Could you check a few things on this drawing? It's one solid part, dimensions in mm from its lowest x, y, z. A direction names the side the tool comes from. Give positions to 0.01 mm unless a question says otherwise; leave off trailing zeros. Loops run counter-clockwise (first coordinate to the right, second up) from the corner with the lowest first, then second, coordinate; pieces in that order, holes last. Notation, with made-up numbers: M 14.5,72.5 L 50.5,72.5 A33 ccw 50.5,106.5 Z; hole C 45.5,86.25 d10. An arc over 180 degrees is marked long. Return JSON: item names as keys, results as strings. Group by question number.
1. If we section it at A-A (z = 7.25): Write out the boundary of the cut face in (x, y), plus the area to 3 significant figures.
2. Please list where these lines run through material, in increasing order: line 1 (X direction, y = 19.5, z = 3.5); line 2 (Y direction, x = 36, z = 5.75); line 3 (Z direction, x = 38.5, y = 3.5).
3. If we mould it in two halves opening along Y, with no side actions, what happens to the marked faces 1, 2, 3 and 4? For each: +Y half, -Y half, draft (parallel to the pull), parting line (faces both ways), or undercut.
4. For the marked faces 5 and 6, which set-ups out of +Z, -Z, +X, -X, +Y, -Y let a thin tool reach every point of the face, with its end or its side?
5. If we section it at C-C (x = 17): Write out the boundary of the cut face in (y, z).
6. If we section it at B-B (y = 13.5): Write out the boundary of the cut face in (x, z).
7. For pin 1 (0.5 mm diameter, centred on x = 63, z = 0.5, fed in from -Y); pin 2 (0.7 mm diameter, centred on x = 63, z = 0, fed in from +Y); pin 3 (0.6 mm diameter, centred on x = 63, y = 15, fed in from -Z), each with a flat end and sliding along its axis, tell me the tip position at first contact or that it passes through.
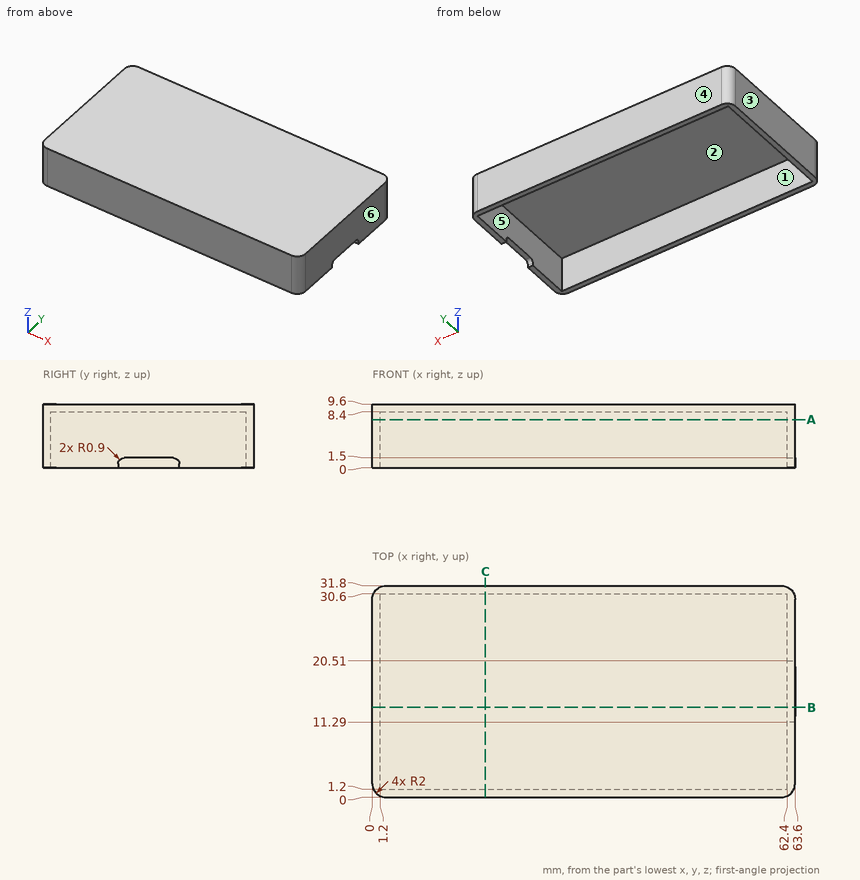
Answer:
{
 "1": {"outline": "M 0,2 A2 ccw 2,0 L 61.6,0 A2 ccw 63.6,2 L 63.6,29.8 A2 ccw 61.6,31.8 L 2,31.8 A2 ccw 0,29.8 Z; hole M 1.2,1.2 L 62.4,1.2 L 62.4,30.6 L 1.2,30.6 Z", "area": "220 mm²"},
 "2": {"line 1": "x = 0 to 1.2, 62.4 to 63.6", "line 2": "y = 0 to 1.2, 30.6 to 31.8", "line 3": "z = 8.4 to 9.6"},
 "3": {"face 1": "undercut", "face 2": "undercut", "face 3": "draft", "face 4": "+Y half"},
 "4": {"face 5": "-Z", "face 6": "+Z, -Z, +X, +Y, -Y"},
 "5": {"outline": "M 0,0 L 1.2,0 L 1.2,8.4 L 30.6,8.4 L 30.6,0 L 31.8,0 L 31.8,9.6 L 0,9.6 Z"},
 "6": {"outline": "M 0,0 L 1.2,0 L 1.2,8.4 L 62.4,8.4 L 62.4,1.5 L 63.6,1.5 L 63.6,9.6 L 0,9.6 Z"},
 "7": {"pin 1": "stops at y = 0.36", "pin 2": "stops at y = 31.5", "pin 3": "stops at z = 1.5"}
}
